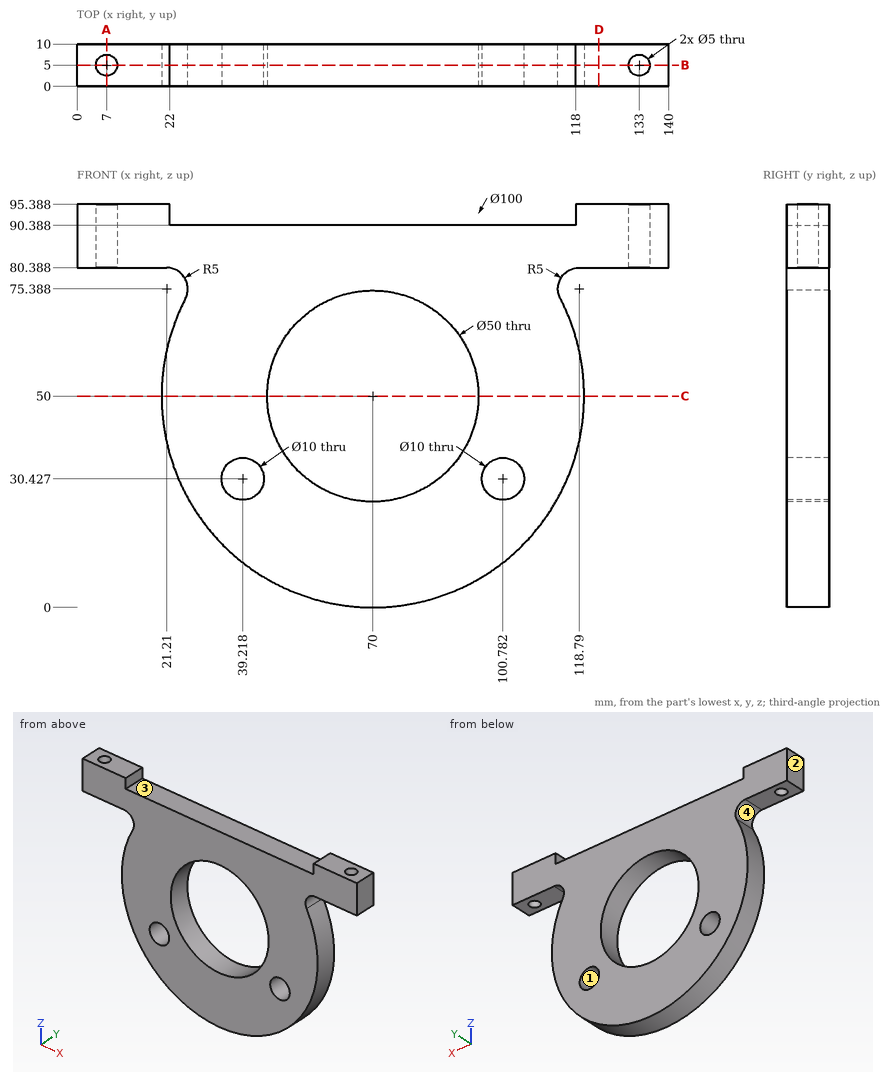
Study the drawing (mm; zero at the part's minimum x, y, z) and answer. Round coordinates to 2 decimals unless told otherwise and drop trailing zeros. Loops run counter-clockwise (first coordinate to the right, second up) from the corner with the lowest first, then second, coordinate; pieces in that order, holes last.
Q1. Section D-D, the plane x = 123.5 is taken. Determine the outline of the cut face in (y, z).
Q2. Section A-A, the plane x = 7 is taken. Determine the outline of the cut face in (y, z).
Q3. Section C-C, the plane z = 50 is taken. Determine the outline of the cut face in (x, y).
Q4. Find the intervals of material crossed by line 1 (X direction, y = 9, z = 91.5); line 2 (X direction, y = 3.5, z = 50); line 3 (Y direction, x = 7, z = 92), in increasing order.
Q5. Section B-B, the plane y = 5 is taken. Determine the outline of the cut face in (x, z) (1 decimal), then the cut area to 3 significant figures.
Q6. For a pull along Z with two mould halves and no side action, classify the marked faces 1, 2, 3 and 4 as released by +Z, released by -Z, zero draft, split by the parting line, or undercut.
Q7. Given pin 1 Ø3 at (y, z) = (1.5, 29) entering from +X; pin 2 Ø1.5 at (y, z) = (2, 42.5) entering from -X; pin 3 Ø1 at (y, z) = (5.5, 46.5) entering from +X; pin 4 Ø4 at (x, y) = (133, 5) entering from -Z, each flat-ended and moving along its own axis, determine where each tip first touches the part or whether it passes through.
Completed:
1. outline: (0, 80.39) - (10, 80.39) - (10, 95.39) - (0, 95.39) - close
2. outline: (0, 80.39) - (2.5, 80.39) - (2.5, 95.39) - (0, 95.39) - close; (7.5, 80.39) - (10, 80.39) - (10, 95.39) - (7.5, 95.39) - close
3. outline: (20, 0) - (45, 0) - (45, 10) - (20, 10) - close; (95, 0) - (120, 0) - (120, 10) - (95, 10) - close
4. line 1: x = 0 to 22, 118 to 140
4. line 2: x = 20 to 45, 95 to 120
4. line 3: y = 0 to 2.5, 7.5 to 10
5. outline: (0, 80.4) - (4.5, 80.4) - (4.5, 95.4) - (0, 95.4) - close; (9.5, 80.4) - (21.2, 80.4) arc R5 cw to (25.6, 73.1) arc R50 ccw (long way) to (114.4, 73.1) arc R5 cw to (118.8, 80.4) - (130.5, 80.4) - (130.5, 95.4) - (118, 95.4) - (118, 90.4) - (22, 90.4) - (22, 95.4) - (9.5, 95.4) - close; (135.5, 80.4) - (140, 80.4) - (140, 95.4) - (135.5, 95.4) - close; hole circle Ø10 at (39.2, 30.4); hole circle Ø50 at (70, 50); hole circle Ø10 at (100.8, 30.4)
5. area: 6,150 mm2
6. face 1: undercut
6. face 2: zero draft
6. face 3: released by +Z
6. face 4: undercut
7. pin 1: stops at x = 116.04
7. pin 2: stops at x = 20.46
7. pin 3: stops at x = 119.91
7. pin 4: passes through
